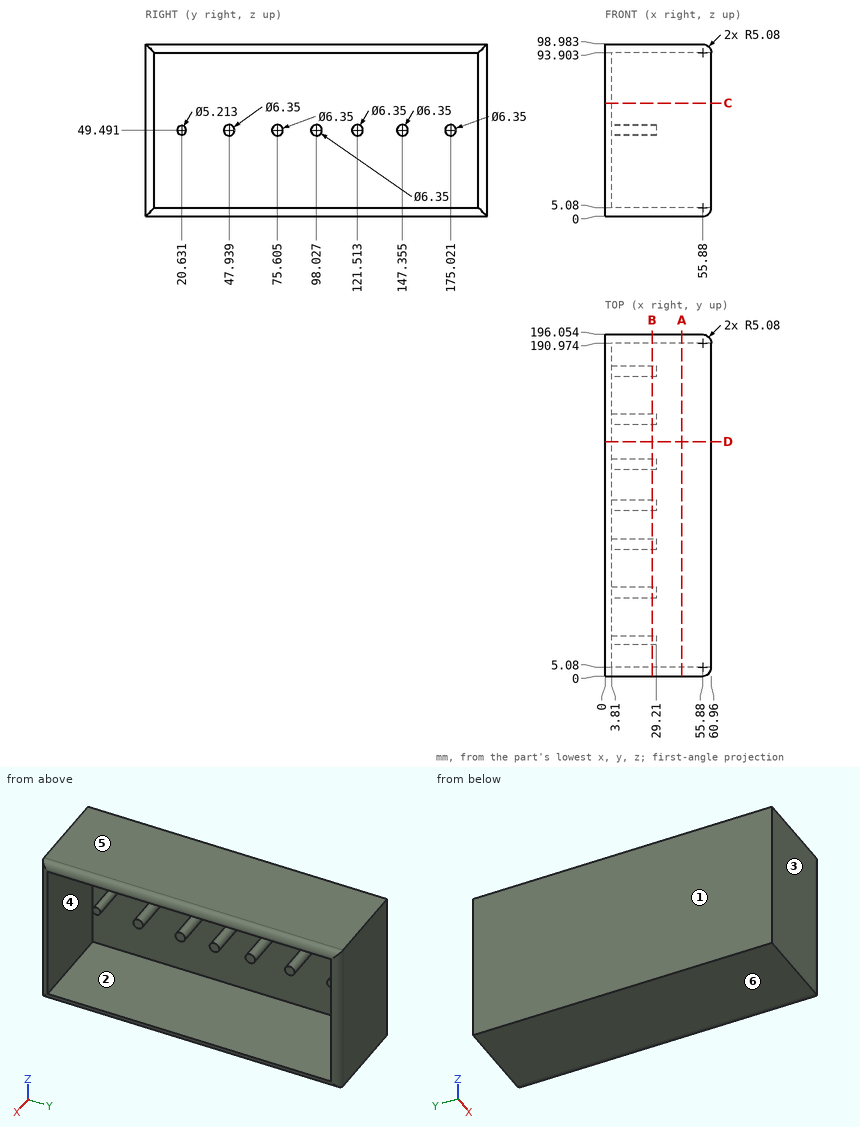
Here's the drawing with two shaded views (mm, measured from the low corner). I have some questions. A direction names the side the tool comes from. Give positions to 0.01 mm unless a question says otherwise; leave off trailing zeros. Write each loop counter-clockwise with the first axis right and the second up, starting at its lowest first coordinate (ties: lowest second). Pieces come first, ordered by that corner, then holes. Notation, with made-up numbers: (-20.75, 61.25) -> (-15.75, 61.25) arc R8 cw to (-15.75, 67.25) -> close; hole circle Ø6 at (-0.5, 48). An arc over 180 degrees is marked (long way). Answer as a JSON object with one key per item and string values. Group by question number.
Item 1: We'd pull the mould along Z, two halves only. Please class the marked faces 3, 4, 5 and 6: +Z half, -Z half, draft (parallel to the pull), parting line (faces both ways), or undercut.
Item 2: For the marked faces 1 and 2, which set-ups out of +Z, -Z, +X, -X, +Y, -Y let a thin tool reach every point of the face, with its end or its side?
Item 3: I'm going to push flat-ended pins straight in: P1, Ø2.5, axis at y = 21.5, z = 49.5, coming from the +X side; P2, Ø5, axis at y = 101.5, z = 72.5, coming from the +X side. Where does each tip first touch, or does it pass through?
Item 4: Suppose I cut it at C-C (z = 65). Please give me the cut outline in (x, y), plus the area to 3 significant figures.
Item 5: Suppose I cut it at B-B (x = 27). State how many separate pieces and enclosed holes the cut face has.
Item 6: Please list where these lines run through material, in increasing order: line 1 (Z direction, x = 41, y = 18.5); line 2 (Y direction, x = 6, z = 59); line 3 (X direction, y = 67.5, z = 46). Write a range as [from, to].
Item 7: Suppose I cut it at D-D (y = 134.5). Please give me the cut outline in (x, z).
Item 8: Suppose I cut it at A-A (x = 44). Please give me the cut outline in (y, z).
Findings:
{
 "1": {"face 3": "draft", "face 4": "undercut", "face 5": "+Z half", "face 6": "-Z half"},
 "2": {"face 1": "+Z, -Z, -X, +Y, -Y", "face 2": "+X"},
 "3": {"P1": "stops at x = 29.21", "P2": "stops at x = 3.81"},
 "4": {"outline": "(0, 0) -> (55.88, 0) arc R5.08 ccw to (60.96, 5.08) -> (3.81, 5.08) -> (3.81, 190.97) -> (60.96, 190.97) arc R5.08 ccw to (55.88, 196.05) -> (0, 196.05) -> close", "area": "1,320 mm²"},
 "5": {"separate pieces": "8", "enclosed holes": "1"},
 "6": {"line 1": "z = [0, 5.08], [93.9, 98.98]", "line 2": "y = [0, 5.08], [190.97, 196.05]", "line 3": "x = [0, 3.81]"},
 "7": {"outline": "(0, 0) -> (55.88, 0) arc R5.08 ccw to (60.96, 5.08) -> (3.81, 5.08) -> (3.81, 93.9) -> (60.96, 93.9) arc R5.08 ccw to (55.88, 98.98) -> (0, 98.98) -> close"},
 "8": {"outline": "(0, 0) -> (196.05, 0) -> (196.05, 98.98) -> (0, 98.98) -> close; hole (5.08, 5.08) -> (190.97, 5.08) -> (190.97, 93.9) -> (5.08, 93.9) -> close"}
}
